Here's how the part is built. I have some questions about the finished solid (model axes, mm). Face numbers are marked on the shaded views. Give positions to 0.01 mm unless a question says otherwise; leave off trailing zeros. Order: outer loops, then holes, each group sorted by start corner. A loop starts at its lowest first (then second) coordinate and runs counter-clockwise, first axis right, second up. Notation, with made-up numbers: M 5,79.5 L 47,79.5 A29 ccw 47,113.5 Z; hole C 47,80 d1. An arc over 180 degrees is marked long. One line per item, written item: value. Start each with the question number.
Autodesk Fusion 360 part; units mm, degrees
sketch "Sketch1" plane through (0, 0, 0) normal (0, 0, 1) x (1, 0, 0)
  line L0 (10, 7.5) -> (-10, 7.5)
  line L1 (-10, 7.5) -> (-10, -7.5)
  line L2 (-10, -7.5) -> (10, -7.5)
  line L3 (10, -7.5) -> (10, 7.5)
  line L4 (10, 7.5) -> (-10, -7.5) construction
  line L5 (-10, 7.5) -> (10, -7.5) construction
  circle A0 centre (0, 0) radius 3.25
  dimension "d1" = 20
  dimension "d2" = 15
  dimension "d3" = 6.5
extrude "Extrude1" add sketch "Sketch1" along normal blind 6.5
chamfer "Chamfer1" distance 4 distance2 4 2 edges at (-10, -7.5, 3.25) (10, -7.5, 3.25) measured on face at (-10, 2.5, 2.1667) measured on face at (-3.3333, -7.5, 4.3333)
chamfer "Chamfer2" distance 2 distance2 2 2 edges at (-8, -5.5, 6.5) (8, -5.5, 6.5) measured on face at (-7.3333, -6.1667, 2.1667) measured on face at (8.6667, -4.8333, 2.1667)
sketch "Sketch2" plane through (0, 0, 6.5) normal (0, 0, 1) x (-1, 0, 0)
  line L0 (-3.1716, 7.5) -> (-10, 0.6716)
  line L1 (-10, 0.6716) -> (-10, -7.5)
  line L2 (-10, -7.5) -> (10, -7.5)
  line L3 (10, -7.5) -> (10, 0.6716)
  line L4 (10, 0.6716) -> (3.1716, 7.5)
  line L5 (3.1716, 7.5) -> (-3.1716, 7.5)
  circle A0 centre (0, 0) radius 3.25
  circle A1 centre (0, 0) radius 5.5
  dimension "d10" = 11
extrude "Extrude2" cut sketch "Sketch2" against normal blind 1 contours A1
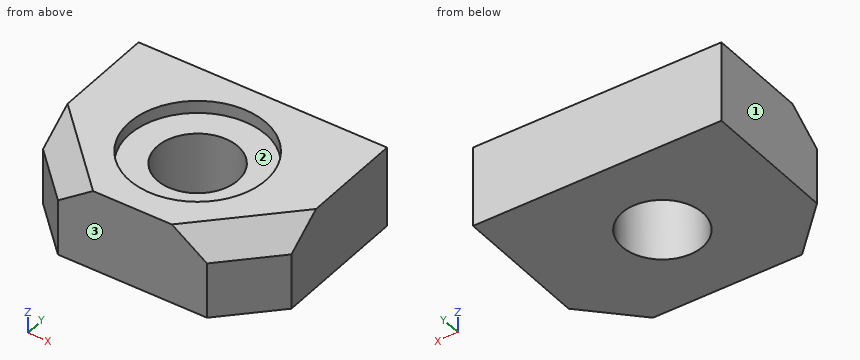
Item 1: We'd pull the mould along X, two halves only. Please class the marked faces 1, 2 and 3: +X half, -X half, draft (parallel to the pull), parting line (faces both ways), or undercut.
Item 2: I want a section at A-A on x = 0. Write out the boundary of the cut face in (y, z).
Item 3: I want a section at B-B on y = 0. Write out the boundary of the cut face in (x, z), plus the area to 4 significant figures.
Item 4: I want a section at C-C on z = 0.5. Write out the boundary of the cut face in (x, y), plus the area to 3 significant figures.
Item 5: I want a section at D-D on x = 4. Write out the boundary of the cut face in (y, z), plus the area to 3 significant figures.
Item 6: Please list where these lines run through material, in increasing order: probe 1 along X at (y, z) = (0, 6.2); probe 2 along Y at (x, z) = (0, 3.8); probe 3 along Y at (x, z) = (0, 5.75). Write a range as [from, to].
Answer below:
1. face 1: -X half
1. face 2: undercut
1. face 3: draft
2. outline: M -7.5,0 L -3.25,0 L -3.25,5.5 L -5.5,5.5 L -5.5,6.5 L -7.5,6.5 Z; M 3.25,0 L 7.5,0 L 7.5,6.5 L 5.5,6.5 L 5.5,5.5 L 3.25,5.5 Z
3. outline: M -10,0 L -3.25,0 L -3.25,5.5 L -5.5,5.5 L -5.5,6.5 L -10,6.5 Z; M 3.25,0 L 10,0 L 10,6.5 L 5.5,6.5 L 5.5,5.5 L 3.25,5.5 Z
3. area: 83.25 mm²
4. outline: M -10,-3.5 L -6,-7.5 L 6,-7.5 L 10,-3.5 L 10,7.5 L -10,7.5 Z; hole C 0,0 d6.5
4. area: 251 mm²
5. outline: M -7.5,0 L 7.5,0 L 7.5,6.5 L 3.77,6.5 L 3.77,5.5 L -3.77,5.5 L -3.77,6.5 L -6.67,6.5 L -7.5,5.91 Z
5. area: 89.7 mm²
6. probe 1: x = [-10, -5.5], [5.5, 10]
6. probe 2: y = [-7.5, -3.25], [3.25, 7.5]
6. probe 3: y = [-7.5, -5.5], [5.5, 7.5]
